from build123d import *

# Parameters (mm, degrees)
BOSS_EXTRUDE1_DEPTH = 3
SKETCH2_R           = 1.5
CUT_EXTRUDE3_DEPTH  = 3
CUT_EXTRUDE4_START  = -10
CUT_EXTRUDE4_DEPTH  = 10
BOSS_EXTRUDE2_START = -3
BOSS_EXTRUDE2_DEPTH = 3
SKETCH5_W           = 0.56
SKETCH5_H           = 32.898596714
CUT_EXTRUDE5_DEPTH  = 3
SKETCH6_W           = 0.2
SKETCH6_H           = 32.898596714
CUT_EXTRUDE6_DEPTH  = 3
SKETCH7_R           = 2
CUT_EXTRUDE8_DEPTH  = 3
BOSS_EXTRUDE3_START = -3
BOSS_EXTRUDE3_DEPTH = 3
CUT_EXTRUDE9_START  = -3
CUT_EXTRUDE9_DEPTH  = 3
BOSS_EXTRUDE5_START = -3
BOSS_EXTRUDE5_DEPTH = 3
CUT_EXTRUDE10_START = -2
CUT_EXTRUDE10_DEPTH = 2
CUT_EXTRUDE11_START = -3
CUT_EXTRUDE11_DEPTH = 3
SKETCH13_R          = 1.5
CUT_EXTRUDE12_DEPTH = 1
CUT_EXTRUDE13_DEPTH = 1
SKETCH16_R          = 1.5
CUT_EXTRUDE16_DEPTH = 10


with BuildPart() as part:
    # Sketch1 → Boss-Extrude1 (new body)
    with BuildSketch(Plane.XY):
        with BuildLine():
            Line((-11, 25.5), (-22.790038711, 29.780264196))
            ThreePointArc((-22.790038711, 29.780264196), (0, -37.5), (22.790038711, 29.780264196))
            Line((22.790038711, 29.780264196), (11, 25.5))
            Line((11, 25.5), (-11, 25.5))
        make_face()
    extrude(amount=BOSS_EXTRUDE1_DEPTH)

    # Sketch2 → Cut-Extrude3 (cut)
    with BuildSketch(Plane.XY.offset(3)):
        with Locations((-25.400000001, 10.496905453)):
            Circle(SKETCH2_R)
        with Locations((-25.399981845, -10.493094547)):
            Circle(SKETCH2_R)
        with Locations(Location((25.399981845, -10.493094547, 0), (0, 0, 180))):
            Circle(SKETCH2_R)
        with Locations(Location((25.400000001, 10.496905453, 0), (0, 0, 180))):
            Circle(SKETCH2_R)
    extrude(amount=-CUT_EXTRUDE3_DEPTH, mode=Mode.SUBTRACT)

    # Sketch3 → Cut-Extrude4 (cut)
    with BuildSketch(Plane.XY.offset(3).offset(CUT_EXTRUDE4_START)):
        with BuildLine():
            Line((-30.76, 21.449298357), (-30.76, -21.449298357))
            ThreePointArc((-30.76, -21.449298357), (-37.5, 0), (-30.76, 21.449298357))
        make_face()
        with BuildLine():
            Line((30.76, 21.449298357), (30.76, -21.449298357))
            ThreePointArc((30.76, -21.449298357), (37.5, 0), (30.76, 21.449298357))
        make_face()
    extrude(amount=CUT_EXTRUDE4_DEPTH, mode=Mode.SUBTRACT)

    # Sketch4 → Boss-Extrude2 (add)
    with BuildSketch(Plane.XY.offset(3).offset(BOSS_EXTRUDE2_START)):
        with BuildLine():
            Line((-30.76, -21.449298357), (-30.76, -16.449298357))
            Line((-30.76, -16.449298357), (-33.699711921, -16.449298357))
            ThreePointArc((-33.699711921, -16.449298357), (-32.32667034, -19.006219634), (-30.76, -21.449298357))
        make_face()
        with BuildLine():
            Line((-33.699711921, 16.449298357), (-30.76, 16.449298357))
            Line((-30.76, 16.449298357), (-30.76, 21.449298357))
            ThreePointArc((-30.76, 21.449298357), (-32.32667034, 19.006219634), (-33.699711921, 16.449298357))
        make_face()
        with BuildLine():
            Line((30.76, 21.449298357), (30.76, 16.449298357))
            Line((30.76, 16.449298357), (33.699711921, 16.449298357))
            ThreePointArc((33.699711921, 16.449298357), (32.32667034, 19.006219634), (30.76, 21.449298357))
        make_face()
        with BuildLine():
            Line((30.76, -16.449298357), (30.76, -21.449298357))
            ThreePointArc((30.76, -21.449298357), (32.32667034, -19.006219634), (33.699711921, -16.449298357))
            Line((33.699711921, -16.449298357), (30.76, -16.449298357))
        make_face()
    extrude(amount=BOSS_EXTRUDE2_DEPTH)

    # Sketch5 → Cut-Extrude5 (cut)
    with BuildSketch(Plane.XY.offset(3)):
        with Locations((-30.48, 0)):
            Rectangle(SKETCH5_W, SKETCH5_H)
        with Locations((30.48, 0)):
            Rectangle(SKETCH5_W, SKETCH5_H)
    extrude(amount=-CUT_EXTRUDE5_DEPTH, mode=Mode.SUBTRACT)

    # Sketch6 → Cut-Extrude6 (cut)
    with BuildSketch(Plane.XY.offset(3)):
        with Locations((-30.1, 0)):
            Rectangle(SKETCH6_W, SKETCH6_H)
        with Locations((30.1, 0)):
            Rectangle(SKETCH6_W, SKETCH6_H)
    extrude(amount=-CUT_EXTRUDE6_DEPTH, mode=Mode.SUBTRACT)

    # Sketch7 → Cut-Extrude8 (cut)
    with BuildSketch(Plane.XY.offset(3)):
        with Locations((-19.15, -21.55)):
            Circle(SKETCH7_R)
        with Locations(Location((19.15, -21.55, 0), (0, 0, 180))):
            Circle(SKETCH7_R)
    extrude(amount=-CUT_EXTRUDE8_DEPTH, mode=Mode.SUBTRACT)

    # Sketch8 → Boss-Extrude3 (add)
    with BuildSketch(Plane.XY.offset(3).offset(BOSS_EXTRUDE3_START)):
        with BuildLine():
            Line((-33.699711921, 16.449298357), (-37.299711921, 16.449298357))
            ThreePointArc((-37.299711921, 16.449298357), (-32.744884003, 23.851322108), (-26.390038711, 29.780264196))
            Line((-26.390038711, 29.780264196), (-22.790038711, 29.780264196))
            ThreePointArc((-22.790038711, 29.780264196), (-29.020710607, 23.749702226), (-33.699711921, 16.449298357))
        make_face()
        with BuildLine():
            Line((33.699711921, 16.449298357), (37.299711921, 16.449298357))
            ThreePointArc((37.299711921, 16.449298357), (32.744884003, 23.851322108), (26.390038711, 29.780264196))
            Line((26.390038711, 29.780264196), (22.790038711, 29.780264196))
            ThreePointArc((22.790038711, 29.780264196), (29.020710607, 23.749702226), (33.699711921, 16.449298357))
        make_face()
    extrude(amount=BOSS_EXTRUDE3_DEPTH)

    # Sketch9 → Cut-Extrude9 (cut)
    with BuildSketch(Plane.XY.offset(3).offset(CUT_EXTRUDE9_START)):
        with BuildLine():
            Line((4.733920151, -37.2), (-4.733920151, -37.2))
            ThreePointArc((-4.733920151, -37.2), (0, -37.5), (4.733920151, -37.2))
        make_face()
    extrude(amount=CUT_EXTRUDE9_DEPTH, mode=Mode.SUBTRACT)

    # Sketch10 → Boss-Extrude5 (add)
    with BuildSketch(Plane.XY.offset(3).offset(BOSS_EXTRUDE5_START)):
        with BuildLine():
            ThreePointArc((-4.733920151, -37.2), (-21.838816892, -30.484685938), (-33.699711921, -16.449298357))
            Line((-33.699711921, -16.449298357), (-37.299711921, -16.449298357))
            ThreePointArc((-37.299711921, -16.449298357), (-23.43831182, -30.624902723), (-4.733920151, -37.2))
        make_face()
        with BuildLine():
            ThreePointArc((33.699711921, -16.449298357), (21.838816892, -30.484685938), (4.733920151, -37.2))
            ThreePointArc((4.733920151, -37.2), (23.43831182, -30.624902723), (37.299711921, -16.449298357))
            Line((37.299711921, -16.449298357), (33.699711921, -16.449298357))
        make_face()
        with BuildLine():
            Line((4.733920151, -37.2), (-4.733920151, -37.2))
            ThreePointArc((-4.733920151, -37.2), (0, -37.457659609), (4.733920151, -37.2))
        make_face()
    extrude(amount=BOSS_EXTRUDE5_DEPTH)

    # Sketch11 → Cut-Extrude10 (cut)
    with BuildSketch(Plane.XY.offset(3).offset(CUT_EXTRUDE10_START)):
        with BuildLine():
            Line((-30, 16.449298357), (-30, 13.449298357))
            Line((-30, 13.449298357), (30, 13.449298357))
            Line((30, 13.449298357), (30, 16.449298357))
            Line((30, 16.449298357), (37.299711921, 16.449298357))
            ThreePointArc((37.299711921, 16.449298357), (32.744884003, 23.851322108), (26.390038711, 29.780264196))
            Line((26.390038711, 29.780264196), (22.790038711, 29.780264196))
            Line((22.790038711, 29.780264196), (11, 25.5))
            Line((11, 25.5), (-11, 25.5))
            Line((-11, 25.5), (-22.790038711, 29.780264196))
            Line((-22.790038711, 29.780264196), (-26.390038711, 29.780264196))
            ThreePointArc((-26.390038711, 29.780264196), (-32.744884003, 23.851322108), (-37.299711921, 16.449298357))
            Line((-37.299711921, 16.449298357), (-30, 16.449298357))
        make_face()
    extrude(amount=CUT_EXTRUDE10_DEPTH, mode=Mode.SUBTRACT)

    # Sketch12 → Cut-Extrude11 (cut)
    with BuildSketch(Plane.XY.offset(3).offset(CUT_EXTRUDE11_START)):
        with BuildLine():
            Line((-30, 13.449298357), (-30, -16.449298357))
            Line((-30, -16.449298357), (-37.299711921, -16.449298357))
            ThreePointArc((-37.299711921, -16.449298357), (0, -37.457659609), (37.299711921, -16.449298357))
            Line((37.299711921, -16.449298357), (30, -16.449298357))
            Line((30, -16.449298357), (30, 13.449298357))
            Line((30, 13.449298357), (-30, 13.449298357))
        make_face()
    extrude(amount=CUT_EXTRUDE11_DEPTH, mode=Mode.SUBTRACT)

    # Sketch13 → Cut-Extrude12 (cut)
    with BuildSketch(Plane.XY.offset(1)):
        with Locations((-28.590038711, 23.780264196)):
            Circle(SKETCH13_R)
        with Locations(Location((28.590038711, 23.780264196, 0), (0, 0, 180))):
            Circle(SKETCH13_R)
    extrude(amount=-CUT_EXTRUDE12_DEPTH, mode=Mode.SUBTRACT)

    # Sketch14 → Cut-Extrude13 (cut)
    with BuildSketch(Plane(origin=(0, 0, 0), x_dir=(-1, 0, 0), z_dir=(0, 0, -1))):
        Polygon((11, 25.5), (11, 13.449298357), (-37.921130539, 13.449298357), (-37.921130539, 32.14037145), (-13.46056527, 32.14037145), (-11, 25.5), align=None)
    extrude(amount=-CUT_EXTRUDE13_DEPTH, mode=Mode.SUBTRACT)

    # Sketch16 → Cut-Extrude16 (cut)
    with BuildSketch(Plane(origin=(0, 0, 0), x_dir=(-1, 0, 0), z_dir=(0, 0, -1))):
        with Locations((16, 20.5)):
            Circle(SKETCH16_R)
    extrude(amount=-CUT_EXTRUDE16_DEPTH, mode=Mode.SUBTRACT)


solid = part.part
Geometry check sheet. Reference: the model listing, model coordinates, mm. A direction names the side the tool comes from. Round coordinates to 2 decimals unless told otherwise and drop trailing zeros. Loops run counter-clockwise (first coordinate to the right, second up) from the corner with the lowest first, then second, coordinate; pieces in that order, holes last.
Item 1: Thickness scan on line 1 (X direction, y = 24.5, z = 0.9); line 2 (Y direction, x = -16, z = 0.75); line 3 (Y direction, x = -15.5, z = 0.3). Record the ranges inside material, lowest first.
Item 2: Cross-section at B-B on z = 0.5. Record the boundary of the cut face in (x, y), then the cut area to 3 significant figures.
Item 3: Access from +Z, -Z, +X, -X, +Y, -Y to the whole of each face (thin tool, end or side, straight path). Record for faces 4 (the flat face through (-30, 14.9, 0.5)), 5 (the flat face through (-11, 19.6, 0.5)).
Item 4: Cross-section at A-A on y = 20.75. Record the boundary of the cut face in (x, z), then the cut area to 3 significant figures.
Item 5: Cross-section at D-D on y = 14.75. Record the boundary of the cut face in (x, z), then the cut area to 3 significant figures.
Item 6: Cross-section at C-C on x = -16.5. Record the boundary of the cut face in (y, z).
Item 7: Mould release check, pull along X, two halves, no side actions. Record for faces 1 (the flat face through (-16.81, 27.61, 0.49)), 2 (the flat face through (-33.6, 16.449, 0.5)), 3 (the cylindrical face through (-30.09, 23.85, 0.51)): pulls with the +X half, pulls with the -X half, needs draft (parallel to the pull), parting line crosses it, or undercut.
Answer sheet:
1. line 1: x = -32.2 to -29.91, -27.27 to -11
1. line 2: y = 13.45 to 19, 22 to 27.32
1. line 3: y = 13.45 to 19.09, 21.91 to 27.13
2. outline: (-37.3, 16.45) - (-30, 16.45) - (-30, 13.45) - (-11, 13.45) - (-11, 25.5) - (-22.79, 29.78) - (-26.39, 29.78) arc R32.48 ccw to start; hole circle Ø3 at (-28.59, 23.78); hole circle Ø3 at (-16, 20.5)
2. area: 309 mm2
3. face 4: +Z, -Z, -X, -Y
3. face 5: +Z, -Z, +X, +Y, -Y
4. outline: (-34.99, 0) - (-17.48, 0) - (-17.48, 1) - (-34.99, 1) - close; (-14.52, 0) - (-11, 0) - (-11, 1) - (-14.52, 1) - close
4. area: 21.0 mm2
5. outline: (-30, 0) - (-11, 0) - (-11, 1) - (-30, 1) - close
5. area: 19.0 mm2
6. outline: (13.45, 0) - (19.09, 0) - (19.09, 1) - (13.45, 1) - close; (21.91, 0) - (27.5, 0) - (27.5, 1) - (21.91, 1) - close
7. face 1: pulls with the +X half
7. face 2: needs draft
7. face 3: undercut
